```python
from build123d import *

# Parameters (mm, degrees)
CROQUIS1_W              = 42
CROQUIS1_H              = 42
SALIENTE_EXTRUIR1_DEPTH = 33
REDONDEO1_R             = 4
CROQUIS2_R              = 11
CROQUIS2_R_2            = 4.75
SALIENTE_EXTRUIR2_DEPTH = 1.5
CROQUIS2_4_R            = 2.5
SALIENTE_EXTRUIR3_DEPTH = 25


with BuildPart() as part:
    # Croquis1 → Saliente-Extruir1 (new body)
    with BuildSketch(Plane.XY):
        Rectangle(CROQUIS1_W, CROQUIS1_H)
    extrude(amount=SALIENTE_EXTRUIR1_DEPTH)

    # Redondeo1
    redondeo1_edges = [part.edges().sort_by_distance(p)[0] for p in [
        (21, -21, 16.5),
        (-21, -21, 16.5),
        (-21, 21, 16.5),
        (21, 21, 16.5),
    ]]
    fillet(redondeo1_edges, radius=REDONDEO1_R)

    # Croquis2 → Saliente-Extruir2 (add)
    with BuildSketch(Plane.XY.offset(33)):
        with Locations(Location((0, 0, 0), (0, 0, 180))):
            Circle(CROQUIS2_R)
        Circle(CROQUIS2_R_2, mode=Mode.SUBTRACT)
    extrude(amount=SALIENTE_EXTRUIR2_DEPTH)

    # Croquis2_4 → Saliente-Extruir3 (add)
    with BuildSketch(Plane.XY.offset(33)):
        with Locations(Location((0, 0, 0), (0, 0, 180))):
            Circle(CROQUIS2_4_R)
    extrude(amount=SALIENTE_EXTRUIR3_DEPTH)


solid = part.part
```
Here's how the part is built. I have some questions about the finished solid (model axes, mm). A direction names the side the tool comes from. Give positions to 0.01 mm unless a question says otherwise; leave off trailing zeros. Order: outer loops, then holes, each group sorted by start corner. A loop starts at its lowest first (then second) coordinate and runs counter-clockwise, first axis right, second up. Notation, with made-up numbers: M 26.25,15 L 78.25,15 A27 ccw 78.25,33 Z; hole C 67,68.25 d7. An arc over 180 degrees is marked long. Use a Markdown table: item, result. Add a question column.
1. For pin 1 Ø3 at (x, y) = (7, 13) entering from +Z; pin 2 Ø10 at (y, z) = (5, 42) entering from -X; pin 3 Ø12.5 at (x, y) = (-8.5, -6) entering from +Z, each with a flat end and sliding along its axis, tell me the tip position at first contact or that it passes through.
2. Suppose I cut it at D-D (y = -8.5). List the corners of the cut face in (x, z) for me, and give its area (3 significant figures).
3. I need wall thicknesses on probe 1 along Y at (x, z) = (0, 34.2); probe 2 along Z at (x, y) = (-16.5, 12.5); probe 3 along Z at (x, y) = (-0.5, -5.5). Which ranges of each line are inside material? Lowest first, please. Write a range as from..to.
4. On a 3-axis mill with a long thin cutter (end or side, diameter ignored), from which of +Z, -Z, +X, -X, +Y, -Y can I reach the whole of each face in a straight line? I mean faces 1 (the flat face through (0, 0, 58)), 2 (the flat face through (2, -2, 33)). Say none if no direction works.
5. Suppose I cut it at A-A (x = 0). List the corners of the cut face in (y, z) for me.
6. If we mould it in two halves opening along X, with no side actions, what happens to faces 3 (the flat face through (0, -21, 16)), 4 (the cylindrical face through (2.192, -4.214, 33.74)), 5 (the cylindrical face through (19.859, 19.797, 16.731))? For each: +X half, -X half, draft (parallel to the pull), parting line (faces both ways), or undercut.
7. Suppose I cut it at C-C (z = 44). List the corners of the cut face in (x, y) for me, and give its area (3 significant figures).
Results list:
| question | item | result |
|---|---|---|
| 1 | pin 1 | stops at z = 33 |
| 1 | pin 2 | stops at x = -2.5 |
| 1 | pin 3 | stops at z = 34.5 |
| 2 | outline | M -21,0 L 21,0 L 21,33 L 6.98,33 L 6.98,34.5 L -6.98,34.5 L -6.98,33 L -21,33 Z |
| 2 | area | 1,410 mm² |
| 3 | probe 1 | y = -11..-4.75, -2.5..2.5, 4.75..11 |
| 3 | probe 2 | z = 0..33 |
| 3 | probe 3 | z = 0..34.5 |
| 4 | face 1 | +Z, +X, -X, +Y, -Y |
| 4 | face 2 | +Z |
| 5 | outline | M -21,0 L 21,0 L 21,33 L 11,33 L 11,34.5 L 4.75,34.5 L 4.75,33 L 2.5,33 L 2.5,58 L -2.5,58 L -2.5,33 L -4.75,33 L -4.75,34.5 L -11,34.5 L -11,33 L -21,33 Z |
| 6 | face 3 | draft |
| 6 | face 4 | undercut |
| 6 | face 5 | +X half |
| 7 | outline | C 0,0 d5 |
| 7 | area | 19.6 mm² |
